Geometry check sheet. Reference: the model listing, model coordinates, mm. A direction names the side the tool comes from. Round coordinates to 2 decimals unless told otherwise and drop trailing zeros. Loops run counter-clockwise (first coordinate to the right, second up) from the corner with the lowest first, then second, coordinate; pieces in that order, holes last. Notation, with made-up numbers: (-25.75, 21.5) - (32.25, 21.5) arc R25 ccw to (32.25, 34.5) - close; hole circle Ø2 at (-5.75, -5). An arc over 180 degrees is marked (long way). Write item = value, one per line.
```python
from build123d import *

# Parameters (mm, degrees)
REVOLVE2_ANGLE           = 7.5
SKETCH4_W                = 33.25
SKETCH4_H                = 13
CUT_EXTRUDE5_DEPTH       = 19
SKETCH7_W                = 33.25
SKETCH7_H                = 13
CUT_EXTRUDE7_DEPTH       = 19
CUT_EXTRUDE11_DEPTH      = 1411.389609827
CUT_EXTRUDE11_DEPTH_BACK = 1411.389609827
SKETCH10_W               = 2135.270707333
SKETCH10_H               = 1606.592084843
SKETCH10_W_2             = 966.47859296
SKETCH10_H_2             = 313.33759653
CUT_EXTRUDE12_DEPTH      = 268.568661532
CUT_EXTRUDE12_DEPTH_BACK = 268.568661532
CUT_EXTRUDE13_DEPTH      = 1057.643677587
CUT_EXTRUDE13_DEPTH_BACK = 1057.643677587
SKETCH14_R               = 2.904277488


with BuildPart() as part:
    # Sketch2 → Revolve2 (revolve)
    with BuildSketch(Plane.XY):
        with BuildLine():
            Line((0, 993.075249624), (0, 990.6))
            ThreePointArc((0, 990.6), (990.6, 0), (0, -990.6))
            Line((0, -990.6), (0, -993.075249624))
            ThreePointArc((0, -993.075249624), (357.30221933, -926.570869107), (666.748724276, -735.965073963))
            Line((666.748724276, -735.965073963), (742.973100692, -735.965073963))
            Line((742.973100692, -735.965073963), (742.973100692, -658.930514596))
            ThreePointArc((742.973100692, -658.930514596), (993.075236283, 0.162783709), (742.757038562, 659.174053709))
            Line((742.757038562, 659.174053709), (742.757038562, 722.715073963))
            Line((742.757038562, 722.715073963), (681.088374063, 722.715073963))
            ThreePointArc((681.088374063, 722.715073963), (366.393230651, 923.013787519), (0, 993.075249624))
        make_face()
    revolve(axis=Axis((0, 993.075249624, 0), (0, -1, 0)), revolution_arc=REVOLVE2_ANGLE)

    # Sketch4 → Cut-Extrude5 (cut)
    with BuildSketch(Plane.XZ.offset(735.965073963)):
        with Locations((705.258501449, 49.061390401)):
            Rectangle(SKETCH4_W, SKETCH4_H)
    extrude(amount=-CUT_EXTRUDE5_DEPTH, mode=Mode.SUBTRACT)

    # Sketch7 → Cut-Extrude7 (cut)
    with BuildSketch(Plane(origin=(0, 722.715073963, 0), x_dir=(-1, 0, 0), z_dir=(0, 1, 0))):
        with Locations((-714.999743141, 46.422731407)):
            Rectangle(SKETCH7_W, SKETCH7_H)
    extrude(amount=-CUT_EXTRUDE7_DEPTH, mode=Mode.SUBTRACT)

    # Sketch10 → Cut-Extrude11 (cut, two sides: drawn at the far end of the back side and taken through both)
    with BuildSketch(Plane.XY.offset(-CUT_EXTRUDE11_DEPTH_BACK)):
        with Locations((557.489585025, 267.498147025)):
            Rectangle(SKETCH10_W, SKETCH10_H)
        with Locations((142.971717026, -995.026755504)):
            Rectangle(SKETCH10_W_2, SKETCH10_H_2)
    extrude(amount=CUT_EXTRUDE11_DEPTH + CUT_EXTRUDE11_DEPTH_BACK, mode=Mode.SUBTRACT)

    # Sketch13 → Cut-Extrude12 (cut, two sides: drawn at the far end of the back side and taken through both)
    with BuildSketch(Plane(origin=(698.790958408, -705.612958968, 0), x_dir=(-0.7105332241790022, -0.7036636535574307, 0), z_dir=(0.7036636535574307, -0.7105332241790022, 0)).offset(-CUT_EXTRUDE12_DEPTH_BACK)):
        with BuildLine():
            Line((-69.681834332, -97.908818451), (-74.241619372, -183.690208107))
            Line((-74.241619372, -183.690208107), (-254.584821077, -153.98925059))
            Line((-254.584821077, -153.98925059), (-254.584821077, 36.219080684))
            Line((-254.584821077, 36.219080684), (-86.443079936, 59.043829873))
            Line((-86.443079936, 59.043829873), (-74.241619372, 0))
            add(Edge.make_bspline(
                [(-74.241619372, 0), (-74.241619372, -16.364172879), (-73.860987213, -32.728340935), (-72.340019213, -65.387598256), (-71.199683881, -81.682677909), (-69.681834332, -97.908818451)],
                knots=[0, 0, 0, 0, 0.5, 0.5, 1, 1, 1, 1], degree=3))
        make_face()
        with BuildLine():
            Line((58.134257499, -86.096803452), (71.382276514, -183.690208107))
            Line((71.382276514, -183.690208107), (231.781280969, -140.799513279))
            Line((231.781280969, -140.799513279), (262.814223376, 47.631455278))
            Line((262.814223376, 47.631455278), (38.648828203, 72.943770658))
            Line((38.648828203, 72.943770658), (54.124752058, 0))
            add(Edge.make_bspline(
                [(54.124752058, 0), (54.124752058, -14.39118635), (54.459503156, -28.782368118), (55.797005676, -57.502130085), (56.799756733, -71.830701127), (58.134257499, -86.096803452)],
                knots=[0, 0, 0, 0, 0.5, 0.5, 1, 1, 1, 1], degree=3))
        make_face()
    extrude(amount=CUT_EXTRUDE12_DEPTH + CUT_EXTRUDE12_DEPTH_BACK, mode=Mode.SUBTRACT)

    # Sketch14 → Cut-Extrude13 (cut, two sides: drawn at the far end of the back side and taken through both)
    with BuildSketch(Plane(origin=(0, 0, 55.561390401), x_dir=(-1, 0, 0), z_dir=(0, 0, -1)).offset(-CUT_EXTRUDE13_DEPTH_BACK)):
        with Locations((-704.851033101, -726.404105815)):
            Circle(SKETCH14_R)
    extrude(amount=CUT_EXTRUDE13_DEPTH + CUT_EXTRUDE13_DEPTH_BACK, mode=Mode.SUBTRACT)


solid = part.part
```
(1) Section check B-B (x = 698). Enter the section's corners in (y, z).
Answers follow:
outline = (-735.97, 0) - (-702.91, 0) arc R702.91 cw to (-696.88, 91.89) - (-735.97, 91.89) - (-735.97, 55.56) - (-716.97, 55.56) - (-716.97, 42.56) - (-735.97, 42.56) - close
(2) Gauge pin test, flat ends, axial feed: pin 1 (5.5 mm diameter, centred on x = 701, y = -731, fed in from +Z); pin 2 (14.5 mm diameter, centred on x = 700.5, z = 48, fed in from -Y); pin 3 (6 mm diameter, centred on x = 703.5, y = -729.5, fed in from +Z); pin 4 (4.5 mm diameter, centred on x = 704.85, y = -726.4, fed in from +Z). Record the tip position at first contact, or that the pin passes through.
Answers follow:
pin_1 = 92.65
pin_2 = -735.97
pin_3 = 93.01
pin_4 = through
(3) Set-up check for faces 4 (the cylindrical face through (741.427, -696.909, 47.913)), 5 (the flat face through (721.884, -727, 49)), 6 (the cylindrical face through (707.156, -728.171, 21.579)): record each of +Z, -Z, +X, -X, +Y, -Y from which the full face is reachable in a straight line by a thin tool's end or side.
Answers follow:
face_4 = +Z, +X, -Y
face_5 = -Y
face_6 = +Z, -Z
(4) Scan lines: L1, parallel to Z at x = 691, y = -725.5; L2, parallel to Z at x = 697, y = -720.5; L3, parallel to Y at x = 708.5, z = 8. Record each from-to range of solid material in increasing order. Write a range as [from, to].
Answers follow:
L1 = [0, 42.56], [55.56, 90.97]
L2 = [0, 42.56], [55.56, 91.76]
L3 = [-735.97, -692.28]
(5) Section check D-D (x = 686.5). Enter the section's corners in (y, z), then the cut area to 3 significant figures.
Answers follow:
outline = (-735.97, 0) - (-714.15, 0) arc R714.15 cw to (-708.41, 90.38) - (-735.97, 90.38) - close
area = 2,140 mm²
(6) Section check C-C (y = -667). Enter the section's corners in (x, z), then the cut area to 3 significant figures.
Answers follow:
outline = (726.13, 95.6) arc R732.39 cw to (732.39, 0) - (742.97, 0) arc R742.97 ccw to (736.62, 96.98) - close
area = 1,020 mm²
(7) Section check A-A (y = -718.5). Enter the section's corners in (x, z).
Answers follow:
outline = (676.11, 89.01) arc R681.94 cw to (681.94, 0) - (742.97, 0) arc R742.97 ccw to (736.62, 96.98) - close; hole (688.63, 42.56) - (721.88, 42.56) - (721.88, 55.56) - (688.63, 55.56) - close
(8) Mould release check, pull along Z, two halves, no side actions. Record for faces 1 (the flat face through (710.859, -706.255, 93.586)), 2 (the flat face through (709, -727, 55.561)), 3 (the flat face through (717, -706, 0)): pulls with the +Z half, pulls with the -Z half, needs draft (parallel to the pull), parting line crosses it, or undercut.
Answers follow:
face_1 = pulls with the +Z half
face_2 = undercut
face_3 = pulls with the -Z half
